For this review, use the dimensioned drawing (mm, ordinates from the lowest corner) and the shaded views. Round coordinates to 2 decimals unless told otherwise and drop trailing zeros. Write each loop counter-clockwise with the first axis right and the second up, starting at its lowest first coordinate (ties: lowest second). Pieces come first, ordered by that corner, then holes.
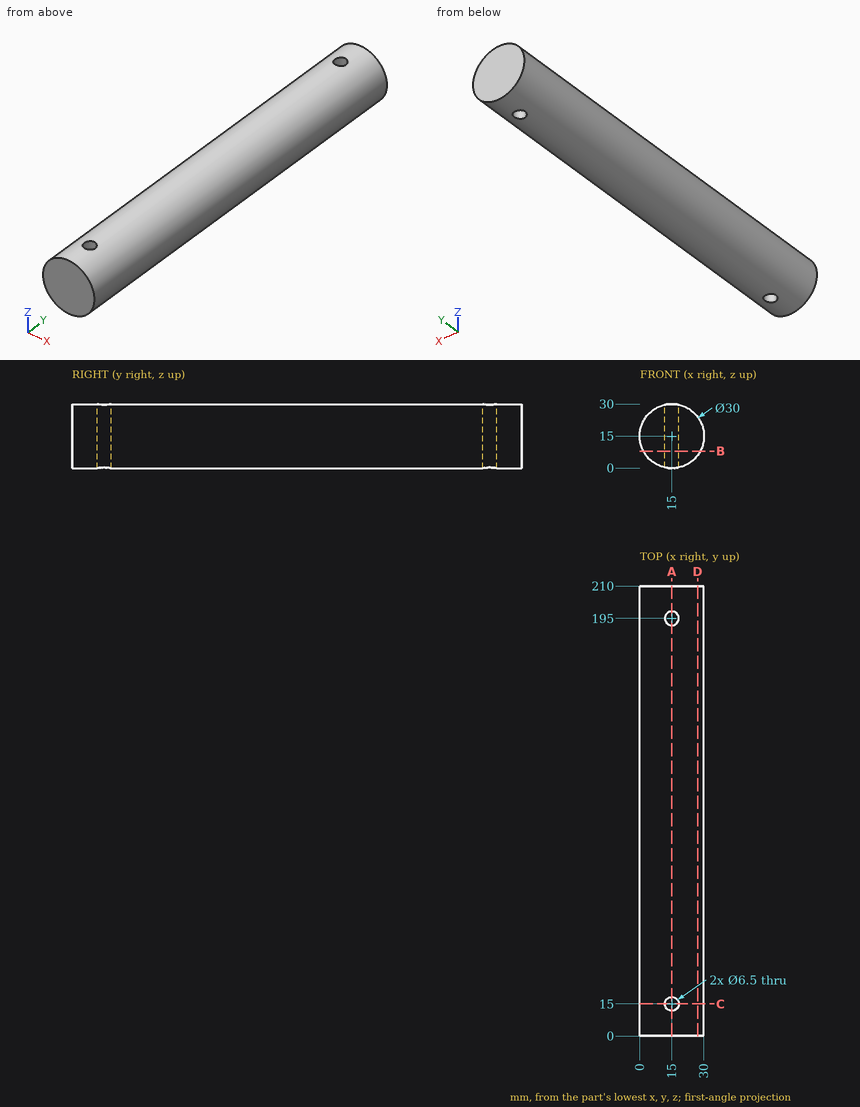
1) For line 1 along Y through (x, z) = (15, 7); line 2 along Y through (x, z) = (12.5, 17); line 3 along X through (y, z) = (188.5, 16), list the stretches that pass through material, from the lowest coordinate up.
2) For P1, Ø4, axis at x = 15, y = 195, coming from the +Z side (3 decimals); P2, Ø6, axis at y = 74, z = 7.5, coming from the -X side; P3, Ø6, axis at y = 168.5, z = 12.5, coming from the +X side; P4, Ø12, axis at x = 21.5, y = 154, coming from the +Z side, all flat-tipped, find the tip position at first contact; note any pin that passes through.
3) Add section C-C on y = 15. State the section outline as (x, z) points, and give its area (3 significant figures).
4) Add section B-B on z = 8. State the section outline as (x, y) points, and give its area (3 significant figures).
5) Add section A-A on x = 15. State the section outline as (y, z) points.
6) Add section D-D on x = 27. State the section outline as (y, z) points.
Computed:
1. line 1: y = 0 to 11.75, 18.25 to 191.75, 198.25 to 210
1. line 2: y = 0 to 12.92, 17.08 to 192.92, 197.08 to 210
1. line 3: x = 0.03 to 29.97
2. P1: passes through
2. P2: stops at x = 0.69
2. P3: stops at x = 30
2. P4: stops at z = 29.99
3. outline: (11.75, 0.36) - (11.75, 29.64) arc R15 ccw to start; (18.25, 0.36) arc R15 ccw to (18.25, 29.64) - close
3. area: 513 mm2
4. outline: (1.73, 0) - (28.27, 0) - (28.27, 210) - (1.73, 210) - close; hole circle Ø6.5 at (15, 15); hole circle Ø6.5 at (15, 195)
4. area: 5,510 mm2
5. outline: (0, 0) - (11.75, 0) - (11.75, 30) - (0, 30) - close; (18.25, 0) - (191.75, 0) - (191.75, 30) - (18.25, 30) - close; (198.25, 0) - (210, 0) - (210, 30) - (198.25, 30) - close
6. outline: (0, 6) - (210, 6) - (210, 24) - (0, 24) - close
